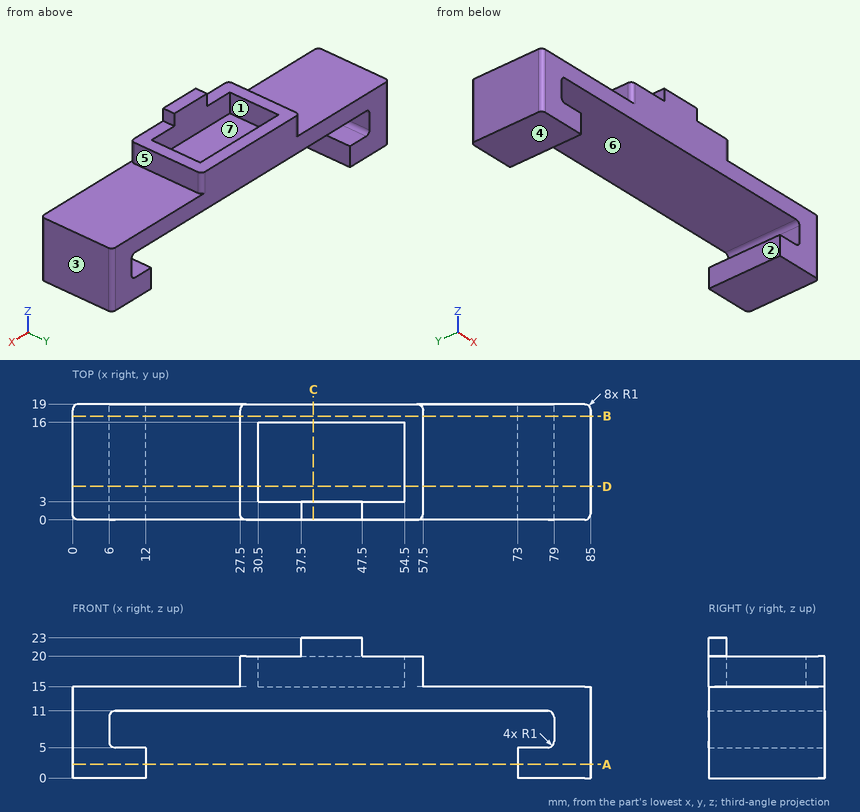
Geometry check sheet. Reference: drawing and pictorial views, mm from the part's lowest x, y, z. A direction names the side the tool comes from. Round coordinates to 2 decimals unless told otherwise and drop trailing zeros. Loops run counter-clockwise (first coordinate to the right, second up) from the corner with the lowest first, then second, coordinate; pieces in that order, holes last. Notation, with made-up numbers: (58, -13) - (74, -13) arc R4 cw to (74, -8) - close; hole circle Ø3 at (86, -35.5). An arc over 180 degrees is marked (long way). Answer in a Markdown table with one row per item. Add a question column.
Q1. Section check D-D on y = 5.5. Enter the section's corners in (x, z).
Q2. Section check B-B on y = 17. Enter the section's corners in (x, z), plus the area to 3 significant figures.
Q3. Material ranges on line 1 (X direction, y = 17, z = 3.5); line 2 (X direction, y = 5.25, z = 15.5); line 3 (X direction, y = 2.5, z = 16.25), recorded low to high.
Q4. Gauge pin test, flat ends, axial feed: pin 1 (2.5 mm diameter, centred on y = 7, z = 17.5, fed in from -X); pin 2 (0.9 mm diameter, centred on y = 1.5, z = 21, fed in from -X); pin 3 (2.5 mm diameter, centred on y = 7, z = 17.5, fed in from +X); pin 4 (1.5 mm diameter, centred on x = 61.5, z = 13, fed in from -Y). Record the tip position at first contact, or that the pin passes through.
Q5. Section check A-A on z = 2.25. Enter the section's corners in (x, y).
Q6. Release check for a two-part mould opening along X. For the marked faces 4, 5, 6 and 7 record: pulls with the +X half, pulls with the -X half, needs draft (parallel to the pull), parting line crosses it, or undercut.
Q7. Section check C-C on x = 39.5. Enter the section's corners in (y, z).
Q8. Tool access check on the marked faces 1, 2 and 3. Record the directions out of +Z, -Z, +X, -X, +Y, -Y that give a thin tool (end or side, any length) a straight path to the whole face; none if there is none.
Found:
| question | item | result |
|---|---|---|
| 1 | outline | (0, 0) - (12, 0) - (12, 5) - (7, 5) arc R1 cw to (6, 6) - (6, 10) arc R1 cw to (7, 11) - (78, 11) arc R1 cw to (79, 10) - (79, 6) arc R1 cw to (78, 5) - (73, 5) - (73, 0) - (85, 0) - (85, 15) - (57.5, 15) - (57.5, 20) - (54.5, 20) - (54.5, 15) - (30.5, 15) - (30.5, 20) - (27.5, 20) - (27.5, 15) - (0, 15) - close |
| 2 | outline | (0, 0) - (12, 0) - (12, 5) - (7, 5) arc R1 cw to (6, 6) - (6, 10) arc R1 cw to (7, 11) - (78, 11) arc R1 cw to (79, 10) - (79, 6) arc R1 cw to (78, 5) - (73, 5) - (73, 0) - (85, 0) - (85, 15) - (57.5, 15) - (57.5, 20) - (27.5, 20) - (27.5, 15) - (0, 15) - close |
| 2 | area | 683 mm² |
| 3 | line 1 | x = 0 to 12, 73 to 85 |
| 3 | line 2 | x = 27.5 to 30.5, 54.5 to 57.5 |
| 3 | line 3 | x = 27.5 to 57.5 |
| 4 | pin 1 | stops at x = 27.5 |
| 4 | pin 2 | stops at x = 37.5 |
| 4 | pin 3 | stops at x = 57.5 |
| 4 | pin 4 | stops at y = 0 |
| 5 | outline | (0, 1) arc R1 ccw to (1, 0) - (12, 0) - (12, 19) - (1, 19) arc R1 ccw to (0, 18) - close; (73, 0) - (84, 0) arc R1 ccw to (85, 1) - (85, 18) arc R1 ccw to (84, 19) - (73, 19) - close |
| 6 | face 4 | needs draft |
| 6 | face 5 | pulls with the +X half |
| 6 | face 6 | undercut |
| 6 | face 7 | undercut |
| 7 | outline | (0, 11) - (19, 11) - (19, 20) - (16, 20) - (16, 15) - (3, 15) - (3, 23) - (0, 23) - close |
| 8 | face 1 | +Z |
| 8 | face 2 | -Z, +Y, -Y |
| 8 | face 3 | +Z, -Z, +X, +Y, -Y |
